Input: part model. Units: mm. Frame: model coordinates. Face numbers are marked on the shaded views. A direction names the side the tool comes from. Round coordinates to 2 decimals unless told otherwise and drop trailing zeros. Write each loop counter-clockwise with the first axis right and the second up, starting at its lowest first coordinate (ties: lowest second). Pieces come first, ordered by that corner, then holes. Notation, with made-up numbers: (26, -13.75) -> (48, -13.75) arc R20 ccw to (48, 17.25) -> close; hole circle Ø8 at (-9, -4). An arc over 180 degrees is marked (long way). Write item = value, one per line. Start each with the question number.
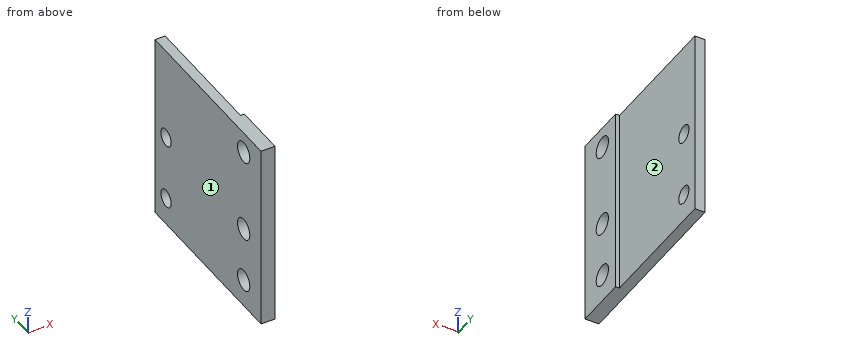
```python
from build123d import *

# Parameters (mm, degrees)
BOSS_EXTRUDE1_DEPTH            = 22
BOSS_EXTRUDE1_DEPTH_BACK       = 5
TAP_DRILL_FOR_M3X0_5_TAP1_D    = 3
TAP_DRILL_FOR_M2_5X0_45_TAP1_D = 2.5


with BuildPart() as part:
    # Sketch1 → Boss-Extrude1 (new, two sides: drawn at the far end of the back side and taken through both)
    with BuildSketch(Plane.XY.offset(-BOSS_EXTRUDE1_DEPTH_BACK)):
        Polygon((0, 0), (2, 0), (2, 7.5), (1.45, 7.5), (1.45, 26), (0, 26), (0, 7.5), align=None)
    extrude(amount=BOSS_EXTRUDE1_DEPTH + BOSS_EXTRUDE1_DEPTH_BACK)

    # Tap Drill for M3x0.5 Tap1 (through all)
    with Locations(Plane(origin=(2, 0, 0), x_dir=(0, 0, -1), z_dir=(1, 0, 0))):
        with Locations((-7, 4.25), (-19, 4.25), (1, 4.25)):
            Hole(TAP_DRILL_FOR_M3X0_5_TAP1_D / 2)

    # Tap Drill for M2.5x0.45 Tap1 (through all)
    with Locations(Plane(origin=(1.45, 0, 0), x_dir=(0, 0, -1), z_dir=(1, 0, 0))):
        with Locations((1, 23.297203827), (-8.5, 23.297203827)):
            Hole(TAP_DRILL_FOR_M2_5X0_45_TAP1_D / 2)


solid = part.part
```
1. Section B-B (y = 4.25). Output: boundary loops of the cut face in (x, z).
2. Section A-A (z = 19). Output: boundary loops of the cut face in (x, y).
3. Line query: line 1 along Y through (x, z) = (0.75, -1); line 2 along Y through (x, z) = (1.55, 7); line 3 along Z through (x, y) = (0.25, 4). Output: solid intervals per line, ascending.
4. Section C-C (z = -1). Output: boundary loops of the cut face in (x, y), then the cut area to 3 significant figures.
5. Pin query (flat end, axial travel): P1, Ø2, axis at y = 23.3, z = 8.5, coming from the -X side; P2, Ø5.5, axis at y = 17.5, z = 3, coming from the +X side. Return the tip coordinate at first contact, or that it passes through.
6. Section D-D (z = 12). Output: boundary loops of the cut face in (x, y).
7. Reachability of the marked faces 1 and 2 from +Z, -Z, +X, -X, +Y, -Y: full face, straight path, thin tool, end or side. Return the list, or none.
Check sheet entries:
q1.outline = (0, -5) -> (2, -5) -> (2, -2.5) -> (0, -2.5) -> close; (0, 0.5) -> (2, 0.5) -> (2, 5.5) -> (0, 5.5) -> close; (0, 8.5) -> (2, 8.5) -> (2, 17.5) -> (0, 17.5) -> close; (0, 20.5) -> (2, 20.5) -> (2, 22) -> (0, 22) -> close
q2.outline = (0, 0) -> (2, 0) -> (2, 2.75) -> (0, 2.75) -> close; (0, 5.75) -> (2, 5.75) -> (2, 7.5) -> (1.45, 7.5) -> (1.45, 26) -> (0, 26) -> close
q3.line_1 = 0 to 2.75, 5.75 to 22.05, 24.55 to 26
q3.line_2 = 0 to 2.75, 5.75 to 7.5
q3.line_3 = -5 to -2.48, 0.48 to 5.52, 8.48 to 17.52, 20.48 to 22
q4.outline = (0, 0) -> (2, 0) -> (2, 2.75) -> (0, 2.75) -> close; (0, 5.75) -> (2, 5.75) -> (2, 7.5) -> (1.45, 7.5) -> (1.45, 22.05) -> (0, 22.05) -> close; (0, 24.55) -> (1.45, 24.55) -> (1.45, 26) -> (0, 26) -> close
q4.area = 32.2 mm2
q5.P1 = through
q5.P2 = 1.45
q6.outline = (0, 0) -> (2, 0) -> (2, 7.5) -> (1.45, 7.5) -> (1.45, 26) -> (0, 26) -> close
q7.face_1 = +Z, -Z, -X, +Y, -Y
q7.face_2 = +Z, -Z, +X, +Y
